Here's how the part is built. I have some questions about the finished solid (model axes, mm). Round coordinates to 2 decimals unless told otherwise and drop trailing zeros. Order: outer loops, then holes, each group sorted by start corner. A loop starts at its lowest first (then second) coordinate and runs counter-clockwise, first axis right, second up. Notation, with made-up numbers: M 66,14 L 122,14 A12 cw 122,34 Z; hole C 50,-29 d10. An arc over 180 degrees is marked long. Write each question's results on one line, items separated by ' | '. Start each with the question number.
```python
from build123d import *

# Parameters (mm, degrees)
SKETCH_1_R      = 4.375
EXTRUDE_1_DEPTH = 5
CHAMFER_1_SIZE  = 1.25


with BuildPart() as part:
    # Эскиз1 → Бобышка-Вытянуть1 (new body)
    with BuildSketch(Plane.XY):
        Polygon((8.5, -4.907477288), (8.5, 4.907477288), (0, 9.814954576), (-8.5, 4.907477288), (-8.5, -4.907477288), (0, -9.814954576), align=None)
        Circle(SKETCH_1_R, mode=Mode.SUBTRACT)
    extrude(amount=EXTRUDE_1_DEPTH)

    # Фаска1
    chamfer_1_edges = [part.edges().sort_by_distance(p)[0] for p in [
        (-4.375, 0, 0),
        (-4.375, 0, 5),
    ]]
    chamfer(chamfer_1_edges, length=CHAMFER_1_SIZE)

    # Эскиз3 → Вырез-Повернуть1 (revolve, cut)
    with BuildSketch(Plane(origin=(0, 0, 0), x_dir=(0, 0, -1), z_dir=(1, 0, 0))):
        Polygon((-0.759189379, 9.814954576), (0, 9.814954576), (0, 8.5), align=None)
        Polygon((-4.240810621, 9.814954576), (-5, 8.5), (-5, 9.814954576), align=None)
    revolve(axis=Axis((0, 0, 0), (0, 0, 1)), mode=Mode.SUBTRACT)


solid = part.part
```
(1) If we mould it in two halves opening along Y, with no side actions, what happens to faces 1 (the flat face through (2, -6, 5)), 2 (the flat face through (4.309, 7.327, 2.465)), 3 (the conical face through (7.627, -4.428, 0.185)), 4 (the cylindrical face through (-3.472, -2.662, 2.482))? For each: pulls with the +Y half, pulls with the -Y half, needs draft (parallel to the pull), parting line crosses it, or undercut.
(2) I want a section at A-A on z = 2.7. Write out the boundary of the cut face in (x, y) (3 decimals), and give its area (3 significant figures).
(3) I'm going to push flat-ended pins straight in: pin 1 Ø2 at (x, z) = (1.5, 2.5) entering from +Y; pin 2 Ø1 at (x, z) = (4, 2.5) entering from +Y; pin 3 Ø2 at (x, y) = (4, -2) entering from +Z. Where does each tip first touch, or does it pass through?
(4) Please list where these lines run through material, in increasing order: line 1 (Y direction, x = -1, z = 3.05); line 2 (Y direction, x = -3.25, z = 3.85); line 3 (X direction, y = 0, z = 3.95) (3 decimals).
Solutions:
1) face 1: needs draft | face 2: pulls with the +Y half | face 3: pulls with the -Y half | face 4: undercut
2) outline: M -8.5,-4.907 L 0,-9.815 L 8.5,-4.907 L 8.5,4.907 L 0,9.815 L -8.5,4.907 Z; hole C 0,0 d8.75 | area: 190 mm^2
3) pin 1: y = 9.53 | pin 2: y = 7.79 | pin 3: z = 4.85
4) line 1: -9.24 to -4.26, 4.26 to 9.24 | line 2: -7.94 to -3.08, 3.08 to 7.94 | line 3: -8.5 to -4.575, 4.575 to 8.5
